Design review of the part shown in the three views and the two pictorial views. Dimensions are in mm from the part's minimum x, y and z. Give positions to 0.01 mm unless a question says otherwise; leave off trailing zeros. Order: outer loops, then holes, each group sorted by start corner. A loop starts at its lowest first (then second) coordinate and runs counter-clockwise, first axis right, second up. Notation, with made-up numbers: (-21, 20) - (24, 20) arc R23 ccw to (24, 49) - close; hole circle Ø3 at (53, -20). An arc over 180 degrees is marked (long way). Put each result on its own line as item: value. Start each with the question number.
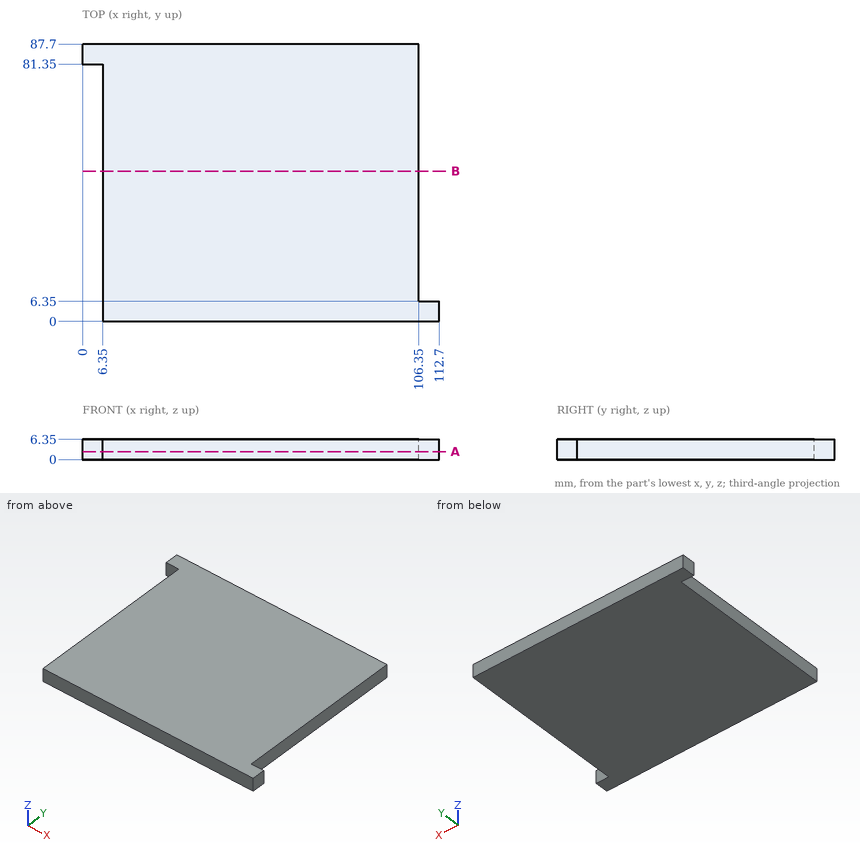
1. Add section B-B, the plane y = 47.5. Give the boundary of the cut face in (x, z), then the cut area to 3 significant figures.
2. Clearance check with flat-ended pins moving along their axes: pin 1 (3 mm diameter, centred on y = 30, z = 3.5, fed in from -X); pin 2 (3 mm diameter, centred on y = 57.5, z = 5, fed in from +X). State where each tip first meets the part, or that it passes through.
3. Wall thickness on line 1 (X direction, y = 24, z = 2.5): over which ranges is the line inside the solid? List them lowest first. Write a range as from..to.
4. Add section A-A, the plane z = 2.5. Give the boundary of the cut face in (x, y).
Found:
1. outline: (6.35, 0) - (106.35, 0) - (106.35, 6.35) - (6.35, 6.35) - close
1. area: 635 mm^2
2. pin 1: stops at x = 6.35
2. pin 2: stops at x = 106.35
3. line 1: x = 6.35..106.35
4. outline: (0, 81.35) - (6.35, 81.35) - (6.35, 0) - (112.7, 0) - (112.7, 6.35) - (106.35, 6.35) - (106.35, 87.7) - (0, 87.7) - close
